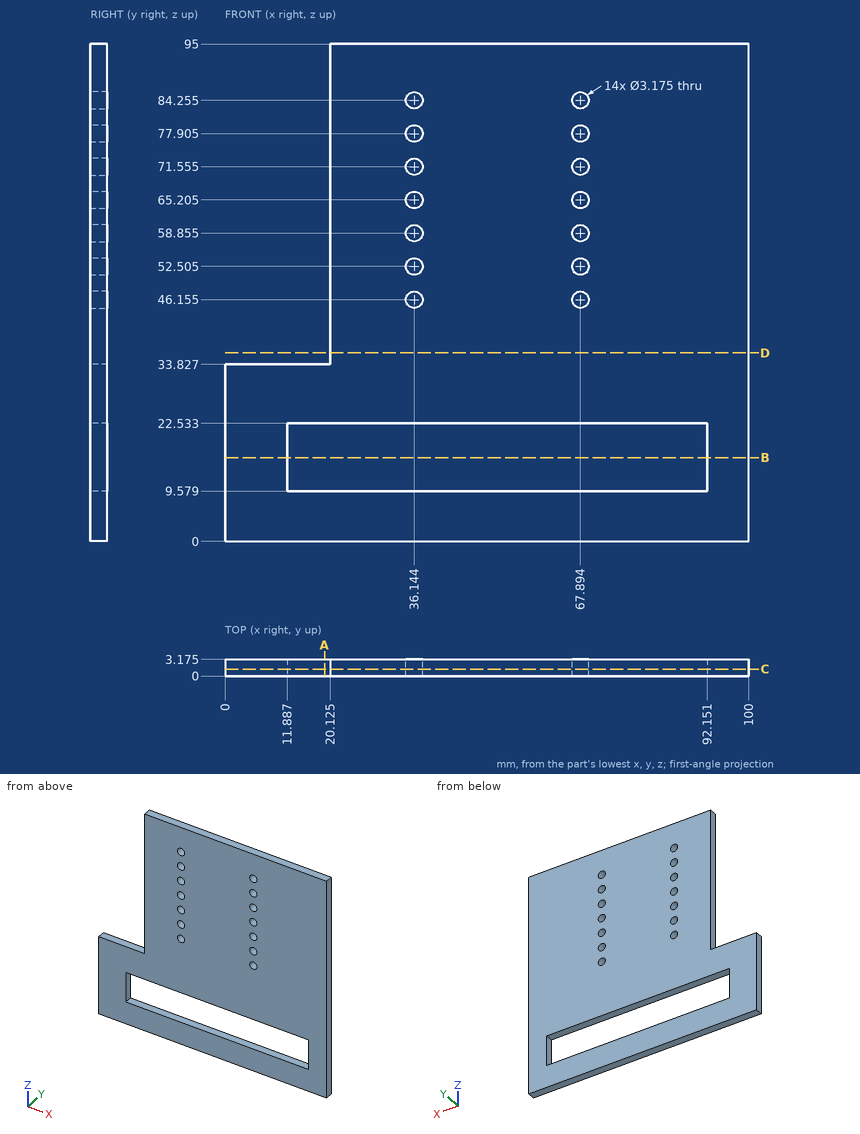
Here's the drawing with two shaded views (mm, measured from the low corner). I have some questions. Coordinates: 2 decimals unless noted, no trailing zeros. Loops run counter-clockwise (first coordinate to the right, second up) from the corner with the lowest first, then second, coordinate; pieces in that order, holes last. Notation, with made-up numbers: (7.5, -32.75) -> (37.5, -32.75) arc R18 ccw to (37.5, -2.75) -> close; hole circle Ø8 at (70.25, -1.5). An arc over 180 degrees is marked (long way). Answer as a JSON object with one key per item and string values.
1) Imagine slicing it at C-C (y = 1.3). Count the separate pieces of the cut face and the enclosed holes in it, then the cut area to 3 significant figures.
Results:
{"separate pieces": "1", "enclosed holes": "15", "area": "7,120 mm^2"}
2) If I drill on line 1 (Z direction, x = 19, y = 0.2); line 2 (Z direction, x = 79.5, y = 1.3); line 3 (X direction, y = 0.7, z = 78) (1 decimal), over which ranges is the centre line in solid material (lowest first)?
Results:
{"line 1": "z = 0 to 9.58, 22.53 to 33.83", "line 2": "z = 0 to 9.58, 22.53 to 95", "line 3": "x = 20.1 to 34.6, 37.7 to 66.3, 69.5 to 100"}
3) Imagine slicing it at A-A (x = 19). Please give me the cut outline in (y, z) (1 decimal).
Results:
{"outline": "(0, 0) -> (3.2, 0) -> (3.2, 9.6) -> (0, 9.6) -> close; (0, 22.5) -> (3.2, 22.5) -> (3.2, 33.8) -> (0, 33.8) -> close"}
4) Imagine slicing it at B-B (z = 16). Please give me the cut outline in (x, y) (1 decimal).
Results:
{"outline": "(0, 0) -> (11.9, 0) -> (11.9, 3.2) -> (0, 3.2) -> close; (92.2, 0) -> (100, 0) -> (100, 3.2) -> (92.2, 3.2) -> close"}
5) Imagine slicing it at D-D (z = 36). Please give me the cut outline in (x, y) (1 decimal).
Results:
{"outline": "(20.1, 0) -> (100, 0) -> (100, 3.2) -> (20.1, 3.2) -> close"}
